Build history of the part. All positions in model axes, mm. Give positions to 0.01 mm unless a question says otherwise; leave off trailing zeros. Loops run counter-clockwise (first coordinate to the right, second up) from the corner with the lowest first, then second, coordinate; pieces in that order, holes last.
1) Flat gauge pin, fed straight in: P1, Ø9.5, axis at x = -50, y = 50, coming from the -Z side. Where does the tip first touch, or does it go through?
2) Two-plate mould, pull along Y, no slides. Class faces 1 (the flat face through (-1, 18, 0)), 2 (the cylindrical face through (-0.672, 22.374, 3.131)), 3 (the flat face through (-1, -75, 3)): +Y half, -Y half, draft (parallel to the pull), parting line (faces both ways), or undercut.
3) Band-saw the part on B-B on z = 3.25. List the corners of the cut face in (x, y).
4) Band-saw the part on A-A on x = -50. List the corners of the cut face in (y, z).
5) Wall check: line 1 (Y direction, x = 50, z = 4.5); line 2 (Y direction, x = 0, z = 2.5); line 3 (X direction, y = -4, z = 6.25). Give the ranges that are in metal, low to high.
6) Band-saw the part on D-D on x = 0. List the corners of the cut face in (y, z), then the cut area to 3 significant figures.
```python
from build123d import *

# Parameters (mm, degrees)
CROQUIS1_W              = 150
CROQUIS1_H              = 150
CROQUIS1_R              = 3.1
CROQUIS1_R_2            = 4.1
CROQUIS1_R_3            = 5
SALIENTE_EXTRUIR1_DEPTH = 6.35


with BuildPart() as part:
    # Croquis1 → Saliente-Extruir1 (new body)
    with BuildSketch(Plane.XY):
        Rectangle(CROQUIS1_W, CROQUIS1_H)
        with Locations((0, 25.4)):
            Circle(CROQUIS1_R, mode=Mode.SUBTRACT)
        with Locations((0, -25.4)):
            Circle(CROQUIS1_R, mode=Mode.SUBTRACT)
        with Locations((-50, 50)):
            Circle(CROQUIS1_R_2, mode=Mode.SUBTRACT)
        with Locations((50, 50)):
            Circle(CROQUIS1_R_2, mode=Mode.SUBTRACT)
        with Locations((50, -50)):
            Circle(CROQUIS1_R_2, mode=Mode.SUBTRACT)
        with Locations((-50, -50)):
            Circle(CROQUIS1_R_2, mode=Mode.SUBTRACT)
        Circle(CROQUIS1_R_3, mode=Mode.SUBTRACT)
    extrude(amount=SALIENTE_EXTRUIR1_DEPTH)


solid = part.part
```
Findings below:
1. P1: stops at z = 0
2. face 1: draft
2. face 2: undercut
2. face 3: -Y half
3. outline: (-75, -75) - (75, -75) - (75, 75) - (-75, 75) - close; hole circle Ø8.2 at (-50, -50); hole circle Ø8.2 at (-50, 50); hole circle Ø10 at (0, 0); hole circle Ø6.2 at (0, -25.4); hole circle Ø6.2 at (0, 25.4); hole circle Ø8.2 at (50, -50); hole circle Ø8.2 at (50, 50)
4. outline: (-75, 0) - (-54.1, 0) - (-54.1, 6.35) - (-75, 6.35) - close; (-45.9, 0) - (45.9, 0) - (45.9, 6.35) - (-45.9, 6.35) - close; (54.1, 0) - (75, 0) - (75, 6.35) - (54.1, 6.35) - close
5. line 1: y = -75 to -54.1, -45.9 to 45.9, 54.1 to 75
5. line 2: y = -75 to -28.5, -22.3 to -5, 5 to 22.3, 28.5 to 75
5. line 3: x = -75 to -3, 3 to 75
6. outline: (-75, 0) - (-28.5, 0) - (-28.5, 6.35) - (-75, 6.35) - close; (-22.3, 0) - (-5, 0) - (-5, 6.35) - (-22.3, 6.35) - close; (5, 0) - (22.3, 0) - (22.3, 6.35) - (5, 6.35) - close; (28.5, 0) - (75, 0) - (75, 6.35) - (28.5, 6.35) - close
6. area: 810 mm2
